Geometry: final body of the model. Coordinates: model frame, mm. Face numbers are marked on the shaded views. A direction names the side the tool comes from. Give positions to 0.01 mm unless a question says otherwise; leave off trailing zeros. Write each loop counter-clockwise with the first axis right and the second up, starting at its lowest first coordinate (ties: lowest second). Pieces come first, ordered by that corner, then holes. Notation, with made-up numbers: M -1,-2 L 44,-2 A15 cw 44,13 Z; hole C -8.75,-7 d5. An arc over 180 degrees is marked long. Use one line per item in the form item = value. Start each with the question number.
Item 1: Material intervals for line 1 along X through (y, z) = (247, 3.1); line 2 along X through (y, z) = (172, 5.5); line 3 along X through (y, z) = (150.5, -1.75), sorted ascending. Write a range as from..to.
Item 2: Section query A-A on y = 157.5. Return loops of the section in (x, z).
Item 3: Pull-direction query (X, two-part tool) for the marked faces 3, 4 and 5; classes: released by +X, released by -X, zero draft, split by the parting line, or undercut.
Item 4: Access query for the marked faces 1 and 2. Directions: +Z, -Z, +X, -X, +Y, -Y. A direction counts if a zero-diameter tool reaches every point of the face in a straight line with its end or side. Return the directions, or none.
Item 5: Contact query for flat-ended pins moving along their axis: P1, Ø3, axis at x = -16, y = 63.5, coming from the -Z side; P2, Ø1, axis at x = -17.5, y = 213.5, coming from the -Z side; P3, Ø4.5, axis at x = -16, y = 49, coming from the -Z side; P4, Ø10, axis at x = 3.5, y = 185.5, coming from the -Z side. Output: stop coordinate, or through.
from build123d import *

# Parameters (mm, degrees)
RUNDUNG_DEPTH                    = 250
SKIZZE2_W                        = 22
SKIZZE2_H                        = 3.270726357
AUSSPARUNGLAUF_DEPTH             = 252.122480077
SKIZZE4_W                        = 20
SKIZZE4_H                        = 87.5
SCHNITT_LINEAR_AUSTRAGEN2_DEPTH  = 252.164667101
SKIZZE5_R                        = 2.4
SCHNITT_LINEAR_AUSTRAGEN4_DEPTH  = 6.4
SKIZZE6_R                        = 2.85
SCHNITT_LINEAR_AUSTRAGEN5_DEPTH  = 1
SKIZZE9_W                        = 35
SKIZZE9_H                        = 6.605082277
SCHNITT_LINEAR_AUSTRAGEN9_DEPTH  = 25
SCHNITT_LINEAR_AUSTRAGEN10_REACH = 228.247
SKIZZE12_R                       = 1.75
SKIZZE14_R                       = 2.4
SCHNITT_LINEAR_AUSTRAGEN11_DEPTH = 6.4
SKIZZE15_R                       = 2.9
SCHNITT_LINEAR_AUSTRAGEN12_DEPTH = 1.2
VERRUNDUNG1_R                    = 5
VERRUNDUNG2_R                    = 1


with BuildPart() as part:
    # Skizze1 → Rundung (new body)
    with BuildSketch(Plane(origin=(0, 0, 0), x_dir=(1, 0, 0), z_dir=(0, 1, 0))):
        with BuildLine():
            Line((-19.158288024, 7.5), (-22.5, 7.5))
            Line((-22.5, 7.5), (-22.5, -7.5))
            Line((-22.5, -7.5), (22.5, -7.5))
            Line((22.5, -7.5), (22.5, 7.5))
            Line((22.5, 7.5), (19.158288024, 7.5))
            ThreePointArc((19.158288024, 7.5), (0, 1.3), (-19.158288024, 7.5))
        make_face()
    extrude(amount=RUNDUNG_DEPTH)

    # Skizze2 → AussparungLauf (cut, through all)
    with BuildSketch(Plane(origin=(0, 250, 0), x_dir=(1, 0, 0), z_dir=(0, 1, 0))):
        with Locations((0, 2.935363178)):
            Rectangle(SKIZZE2_W, SKIZZE2_H)
    extrude(amount=-AUSSPARUNGLAUF_DEPTH, mode=Mode.SUBTRACT)

    # Skizze4 → Schnitt-Linear austragen2 (cut, through all)
    with BuildSketch(Plane(origin=(0, 0, -1.3), x_dir=(-1, 0, 0), z_dir=(0, 0, -1))):
        with Locations((0, 73.75)):
            Rectangle(SKIZZE4_W, SKIZZE4_H)
        with Locations((0, 176.25)):
            Rectangle(SKIZZE4_W, SKIZZE4_H)
    extrude(amount=-SCHNITT_LINEAR_AUSTRAGEN2_DEPTH, mode=Mode.SUBTRACT)

    # Skizze5 → Schnitt-Linear austragen4 (cut)
    with BuildSketch(Plane.XY.offset(7.5)):
        with Locations((-16, 32)):
            Circle(SKIZZE5_R)
        with Locations((16, 32)):
            Circle(SKIZZE5_R)
        with Locations((16, 48)):
            Circle(SKIZZE5_R)
        with Locations((16, 64)):
            Circle(SKIZZE5_R)
        with Locations((16, 80)):
            Circle(SKIZZE5_R)
        with Locations((-16, 48)):
            Circle(SKIZZE5_R)
        with Locations((-16, 64)):
            Circle(SKIZZE5_R)
        with Locations((-16, 80)):
            Circle(SKIZZE5_R)
    extrude(amount=-SCHNITT_LINEAR_AUSTRAGEN4_DEPTH, mode=Mode.SUBTRACT)

    # Skizze6 → Schnitt-Linear austragen5 (cut)
    with BuildSketch(Plane.XY.offset(1.1)):
        with Locations((-16, 32)):
            Circle(SKIZZE6_R)
        with Locations((16, 32)):
            Circle(SKIZZE6_R)
        with Locations((16, 48)):
            Circle(SKIZZE6_R)
        with Locations((16, 64)):
            Circle(SKIZZE6_R)
        with Locations((16, 80)):
            Circle(SKIZZE6_R)
        with Locations((-16, 48)):
            Circle(SKIZZE6_R)
        with Locations((-16, 64)):
            Circle(SKIZZE6_R)
        with Locations((-16, 80)):
            Circle(SKIZZE6_R)
    extrude(amount=-SCHNITT_LINEAR_AUSTRAGEN5_DEPTH, mode=Mode.SUBTRACT)

    # Skizze9 → Schnitt-Linear austragen9 (cut)
    with BuildSketch(Plane.XZ):
        with Locations((0, 4.197458862)):
            Rectangle(SKIZZE9_W, SKIZZE9_H)
    extrude(amount=-SCHNITT_LINEAR_AUSTRAGEN9_DEPTH, mode=Mode.SUBTRACT)

    # Skizze12 → Schnitt-Linear austragen10 (cut, up to next)
    with BuildSketch(Plane.XZ.offset(-25), mode=Mode.PRIVATE) as schnitt_linear_austragen10_sk1:
        with Locations(Location((-5, 4.197458861, 0), (0, 0, 270))):
            Circle(SKIZZE12_R)
    schnitt_linear_austragen10_tool1 = extrude(schnitt_linear_austragen10_sk1.sketch, amount=-SCHNITT_LINEAR_AUSTRAGEN10_REACH, mode=Mode.PRIVATE) & part.part
    # Skizze12 → Schnitt-Linear austragen10 (cut, up to next)
    with BuildSketch(Plane.XZ.offset(-25), mode=Mode.PRIVATE) as schnitt_linear_austragen10_sk2:
        with Locations(Location((5, 4.197458861, 0), (0, 0, 270))):
            Circle(SKIZZE12_R)
    schnitt_linear_austragen10_tool2 = extrude(schnitt_linear_austragen10_sk2.sketch, amount=-SCHNITT_LINEAR_AUSTRAGEN10_REACH, mode=Mode.PRIVATE) & part.part
    add(schnitt_linear_austragen10_tool1.solids().sort_by_distance((-5, 25, 4.197459))[0], mode=Mode.SUBTRACT)
    add(schnitt_linear_austragen10_tool2.solids().sort_by_distance((5, 25, 4.197459))[0], mode=Mode.SUBTRACT)

    # Skizze14 → Schnitt-Linear austragen11 (cut)
    with BuildSketch(Plane(origin=(0, 250, 0), x_dir=(1, 0, 0), z_dir=(0, 1, 0))):
        with Locations(Location((-16, -3.1, 0), (0, 0, 270))):
            Circle(SKIZZE14_R)
        with Locations(Location((16, -3.1, 0), (0, 0, 90))):
            Circle(SKIZZE14_R)
    extrude(amount=-SCHNITT_LINEAR_AUSTRAGEN11_DEPTH, mode=Mode.SUBTRACT)

    # Skizze15 → Schnitt-Linear austragen12 (cut)
    with BuildSketch(Plane(origin=(0, 243.6, 0), x_dir=(1, 0, 0), z_dir=(0, 1, 0))):
        with Locations(Location((-16, -3.1, 0), (0, 0, 270))):
            Circle(SKIZZE15_R)
        with Locations(Location((16, -3.1, 0), (0, 0, 90))):
            Circle(SKIZZE15_R)
    extrude(amount=-SCHNITT_LINEAR_AUSTRAGEN12_DEPTH, mode=Mode.SUBTRACT)

    # Verrundung1
    # the kernel refuses this fillet: 5 mm, written as the material it adds along each edge
    with BuildSketch(Plane(origin=(10, 132.5, -1.3), x_dir=(0, 1, 0), z_dir=(0, 0, 1)), Plane(origin=(-10, 132.5, -1.3), x_dir=(1, 0, 0), z_dir=(0, 0, 1))) as verrundung1_piece_1:
        with BuildLine():
            CenterArc((VERRUNDUNG1_R, VERRUNDUNG1_R), VERRUNDUNG1_R, 180, 90)
            Line((0, VERRUNDUNG1_R), (0, 0))
            Line((0, 0), (VERRUNDUNG1_R, 0))
        make_face()
    extrude(amount=8.8)
    with BuildSketch(Plane(origin=(10, 220, -1.3), x_dir=(0, -1, 0), z_dir=(0, 0, 1)), Plane(origin=(-10, 220, -1.3), x_dir=(1, 0, 0), z_dir=(0, 0, 1)), Plane(origin=(10, 117.5, -1.3), x_dir=(0, -1, 0), z_dir=(0, 0, 1)), Plane(origin=(-10, 117.5, -1.3), x_dir=(1, 0, 0), z_dir=(0, 0, 1))) as verrundung1_piece_2:
        with BuildLine():
            CenterArc((VERRUNDUNG1_R, -VERRUNDUNG1_R), VERRUNDUNG1_R, 90, 90)
            Line((0, -VERRUNDUNG1_R), (0, 0))
            Line((0, 0), (VERRUNDUNG1_R, 0))
        make_face()
    extrude(amount=8.8)
    with BuildSketch(Plane(origin=(10, 30, -1.3), x_dir=(0, 1, 0), z_dir=(0, 0, 1))) as verrundung1_piece_3_section:
        with BuildLine():
            CenterArc((VERRUNDUNG1_R, VERRUNDUNG1_R), VERRUNDUNG1_R, 180, 90)
            Line((0, VERRUNDUNG1_R), (0, 0))
            Line((0, 0), (VERRUNDUNG1_R, 0))
        make_face()
    verrundung1_piece_3 = extrude(amount=8.8, mode=Mode.PRIVATE)
    verrundung1_piece_3 = verrundung1_piece_3 - Plane(origin=(5, 31.149403534, 4.197458861), x_dir=(0, 0, -1), z_dir=(0, -1, 0)) * Cylinder(1.75, 38, mode=Mode.PRIVATE)
    add(verrundung1_piece_3)
    with BuildSketch(Plane(origin=(-10, 30, -1.3), x_dir=(1, 0, 0), z_dir=(0, 0, 1))) as verrundung1_piece_4_section:
        with BuildLine():
            CenterArc((VERRUNDUNG1_R, VERRUNDUNG1_R), VERRUNDUNG1_R, 180, 90)
            Line((0, VERRUNDUNG1_R), (0, 0))
            Line((0, 0), (VERRUNDUNG1_R, 0))
        make_face()
    verrundung1_piece_4 = extrude(amount=8.8, mode=Mode.PRIVATE)
    verrundung1_piece_4 = verrundung1_piece_4 - Plane(origin=(-5, 31.149403677, 4.197458861), x_dir=(0, 0, -1), z_dir=(0, -1, 0)) * Cylinder(1.75, 38, mode=Mode.PRIVATE)
    add(verrundung1_piece_4)

    # Verrundung2
    verrundung2_edges = [part.edges().sort_by_distance(p)[0] for p in [
        (22.5, 125, -7.5),
        (-22.5, 125, -7.5),
    ]]
    fillet(verrundung2_edges, radius=VERRUNDUNG2_R)


solid = part.part
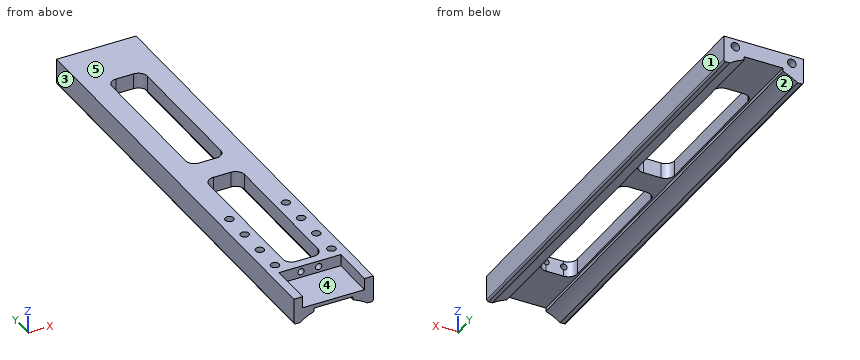
Answer sheet:
q1.line_1 = -22.5..-18.4, -13.6..13.6, 18.4..22.5
q1.line_2 = -22.5..-10, 10..22.5
q1.line_3 = -22.5..-11, 11..22.5
q2.outline = M -22.5,-6.5 A1 ccw -21.5,-7.5 L -19.16,-7.5 A32.7 cw -11,-3.21 L -11,-1.3 L -10,-1.3 L -10,7.5 L -22.5,7.5 Z; M 10,-1.3 L 11,-1.3 L 11,-3.21 A32.7 cw 19.16,-7.5 L 21.5,-7.5 A1 ccw 22.5,-6.5 L 22.5,7.5 L 10,7.5 Z
q3.face_3 = released by -X
q3.face_4 = undercut
q3.face_5 = zero draft
q4.face_1 = +Z, -Z, +X, +Y, -Y
q4.face_2 = -Z, +Y, -Y
q5.P1 = -6.38
q5.P2 = -6.7
q5.P3 = -6.87
q5.P4 = through
